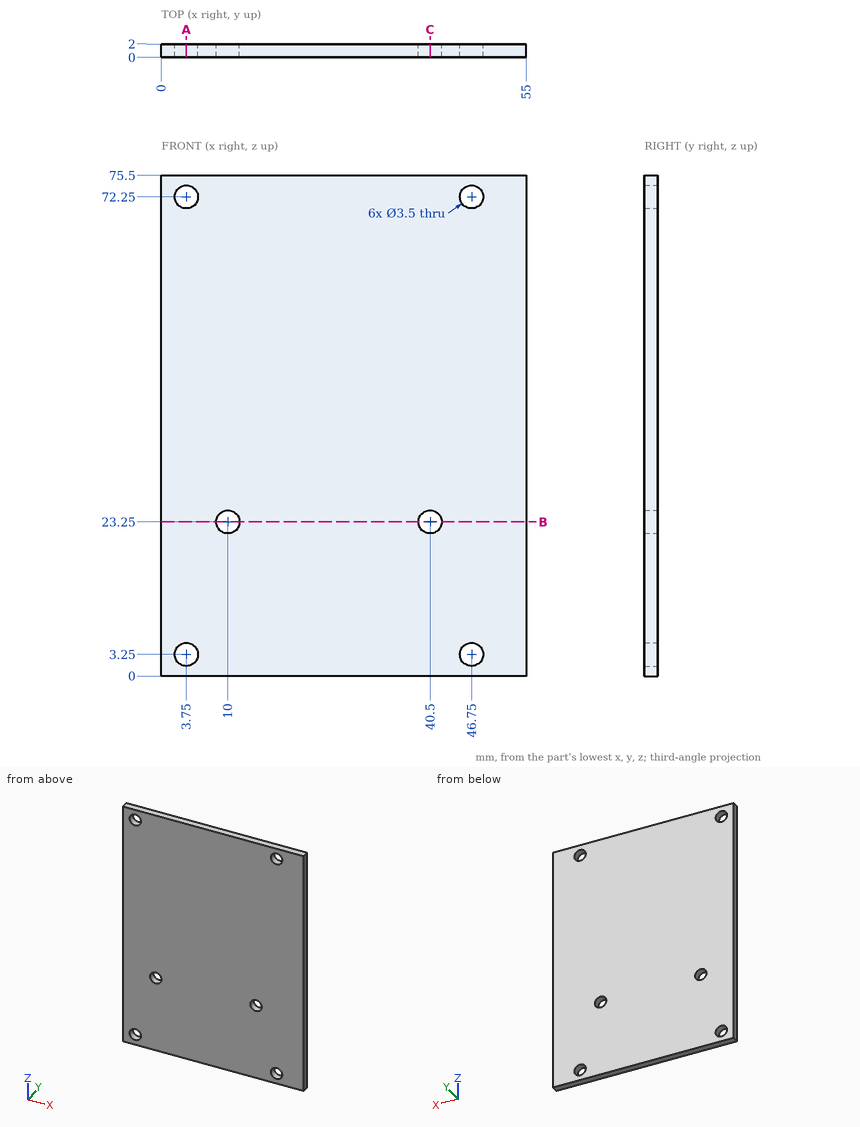
The figure shows three views and two pictorial views of one solid part (mm, origin at its lowest corner). Answer the questions. Give positions to 0.01 mm unless a question says otherwise; leave off trailing zeros. Write each loop counter-clockwise with the first axis right and the second up, starting at its lowest first coordinate (ties: lowest second). Pieces come first, ordered by that corner, then holes.
Q1. The part is cut by section B-B on z = 23.25. Give the vertices of the cut face in (x, y).
Answer:
outline: (0, 0) - (8.25, 0) - (8.25, 2) - (0, 2) - close; (11.75, 0) - (38.75, 0) - (38.75, 2) - (11.75, 2) - close; (42.25, 0) - (55, 0) - (55, 2) - (42.25, 2) - close
Q2. Straight lines are drawn through the part: L1, parallel to Z at x = 46.75, y = 1; L2, parallel to X at y = 1.4, z = 23.25; L3, parallel to X at y = 0.6, z = 72.25. For each, find the intervals that lie inside material, in ascending order.
Answer:
L1: z = 0 to 1.5, 5 to 70.5, 74 to 75.5
L2: x = 0 to 8.25, 11.75 to 38.75, 42.25 to 55
L3: x = 0 to 2, 5.5 to 45, 48.5 to 55
Q3. The part is cut by section A-A on x = 3.75. Give the vertices of the cut face in (y, z), and give its area (3 significant figures).
Answer:
outline: (0, 0) - (2, 0) - (2, 1.5) - (0, 1.5) - close; (0, 5) - (2, 5) - (2, 70.5) - (0, 70.5) - close; (0, 74) - (2, 74) - (2, 75.5) - (0, 75.5) - close
area: 137 mm2
Q4. The part is cut by section C-C on x = 40.5. Give the vertices of the cut face in (y, z), and give its area (3 significant figures).
Answer:
outline: (0, 0) - (2, 0) - (2, 21.5) - (0, 21.5) - close; (0, 25) - (2, 25) - (2, 75.5) - (0, 75.5) - close
area: 144 mm2
